```python
from build123d import *

# Parameters (mm, degrees)
SKETCH_R        = 3.2
SKETCH_R_2      = 7.5
SKETCH_R_3      = 4
PAD_DEPTH       = 8
SKETCH001_R     = 8.6
POCKET_DEPTH    = 6
POCKET001_DEPTH = 8.001


with BuildPart() as part:
    # Sketch → Pad (new body)
    with BuildSketch(Plane.XY):
        with BuildLine():
            ThreePointArc((-32.45, 8.988743), (-41, 0), (-32.45, -8.988743))
            Line((-32.45, -8.988743), (-0.53, -10.586742))
            ThreePointArc((-0.53, -10.586742), (10.6, 0), (-0.53, 10.586742))
            Line((-32.45, 8.988743), (-0.53, 10.586742))
        make_face()
        with Locations((-32, 0)):
            Circle(SKETCH_R, mode=Mode.SUBTRACT)
        Circle(SKETCH_R_2, mode=Mode.SUBTRACT)
        with Locations((-16, 0)):
            Circle(SKETCH_R_3, mode=Mode.SUBTRACT)
    extrude(amount=PAD_DEPTH)

    # Sketch001 → Pocket (cut)
    with BuildSketch(Plane(origin=(0, 0, 0), x_dir=(1, 0, 0), z_dir=(0, 0, -1))):
        Circle(SKETCH001_R)
    extrude(amount=-POCKET_DEPTH, mode=Mode.SUBTRACT)

    # Sketch002 → Pocket001 (cut, through all)
    with BuildSketch(Plane(origin=(0, 0, 0), x_dir=(1, 0, 0), z_dir=(0, 0, -1))):
        Polygon((-34.829016, 4.9), (-37.658033, 0), (-34.829016, -4.9), (-29.170984, -4.9), (-26.341967, 0), (-29.170984, 4.9), align=None)
    extrude(amount=-POCKET001_DEPTH, mode=Mode.SUBTRACT)


solid = part.part
```
Can you work these out from the model? Positions are in its coordinate system, mm. A direction names the side the tool comes from. Round coordinates to 2 decimals unless told otherwise and drop trailing zeros. Loops run counter-clockwise (first coordinate to the right, second up) from the corner with the lowest first, then second, coordinate; pieces in that order, holes last. Notation, with made-up numbers: M 62.5,3 L 90.5,3 A24 ccw 90.5,30 Z; hole C -27.75,58.25 d8. An arc over 180 degrees is marked long. Write item = value, one per line. Start each with the question number.
(1) Which directions (+Z, -Z, +X, -X, +Y, -Y) give clear straight access to the entire face, cutting with the end or side of a thin tool? Please do faces 1 (the face through (-27.74, -2.42, 3.94)), 2 (the face through (1, -8, 6)), 3 (the face through (-16.713, -9.777, 3.944)).
(2) Suppose I cut it at A-A on x = 0. Write out the boundary of the cut face in (y, z).
(3) I'm going to push flat-ended pins straight in: P1, Ø4.5, axis at x = -31, z = 2.5, coming from the -Y side; P2, Ø1, axis at x = 4.5, z = 5.5, coming from the -Y side; P3, Ø4, axis at x = -10.5, z = 4, coming from the -Y side. Where does each tip first touch, or does it pass through?
(4) Suppose I cut it at D-D on y = 6. Write out the boundary of the cut face in (x, z).
(5) Suppose I cut it at B-B on z = 1.25. Write out the boundary of the cut face in (x, y).
(6) If we mould it in two halves opening along Y, with no side actions, what happens to faces 4 (the face through (-21, 0, 0)), 5 (the face through (10.6, -0.2, 3.9)), 6 (the face through (-8.59, -0.38, 2.96))? For each: released by +Y, released by -Y, zero draft, split by the parting line, or undercut.
(7) Suppose I cut it at C-C on y = -3. Write out the boundary of the cut face in (x, z).
(8) I need wall thicknesses on line 1 along X through (y, z) = (-2.5, 4.75); line 2 along X through (y, z) = (1.5, 4.5); line 3 along Y through (x, z) = (0, 6.95). Which ranges of each line are inside material? Lowest first, please.
Answer block:
q1.face_1 = +Z, -Z
q1.face_2 = -Z
q1.face_3 = +Z, -Z, -X, -Y
q2.outline = M -10.6,0 L -8.6,0 L -8.6,6 L -7.5,6 L -7.5,8 L -10.6,8 Z; M 7.5,6 L 8.6,6 L 8.6,0 L 10.6,0 L 10.6,8 L 7.5,8 Z
q3.P1 = -9.17
q3.P2 = -9.82
q3.P3 = -10.19
q4.outline = M -38.71,0 L -6.16,0 L -6.16,6 L -4.5,6 L -4.5,8 L -38.71,8 Z; M 4.5,6 L 6.16,6 L 6.16,0 L 8.74,0 L 8.74,8 L 4.5,8 Z
q5.outline = M -32.45,-8.99 L -0.53,-10.59 A10.6 ccw long -0.53,10.59 L -32.45,8.99 A9 ccw Z; hole M -37.66,0 L -34.83,-4.9 L -29.17,-4.9 L -26.34,0 L -29.17,4.9 L -34.83,4.9 Z; hole C -16,0 d8; hole C 0,0 d17.2
q6.face_4 = zero draft
q6.face_5 = split by the parting line
q6.face_6 = undercut
q7.outline = M -40.49,0 L -35.93,0 L -35.93,8 L -40.49,8 Z; M -28.07,0 L -18.65,0 L -18.65,8 L -28.07,8 Z; M -13.35,0 L -8.06,0 L -8.06,6 L -6.87,6 L -6.87,8 L -13.35,8 Z; M 6.87,6 L 8.06,6 L 8.06,0 L 10.17,0 L 10.17,8 L 6.87,8 Z
q8.line_1 = -40.65 to -36.21, -27.79 to -19.12, -12.88 to -8.23, 8.23 to 10.3
q8.line_2 = -40.87 to -36.79, -27.21 to -19.71, -12.29 to -8.47, 8.47 to 10.49
q8.line_3 = -10.6 to -7.5, 7.5 to 10.6
